Can you work these out from the drawing? Everything is in mm from the part's minimum corner. A direction names the side the tool comes from. Coordinates: 2 decimals unless noted, no trailing zeros. Write each loop counter-clockwise with the first axis right and the second up, starting at its lowest first coordinate (ties: lowest second). Pieces come first, ordered by that corner, then holes. Notation, with made-up numbers: M 11,79 L 16,79 A21 ccw 16,113 Z; hole C 56,56.5 d7. An arc over 180 degrees is marked long. Write item = value, one per line.
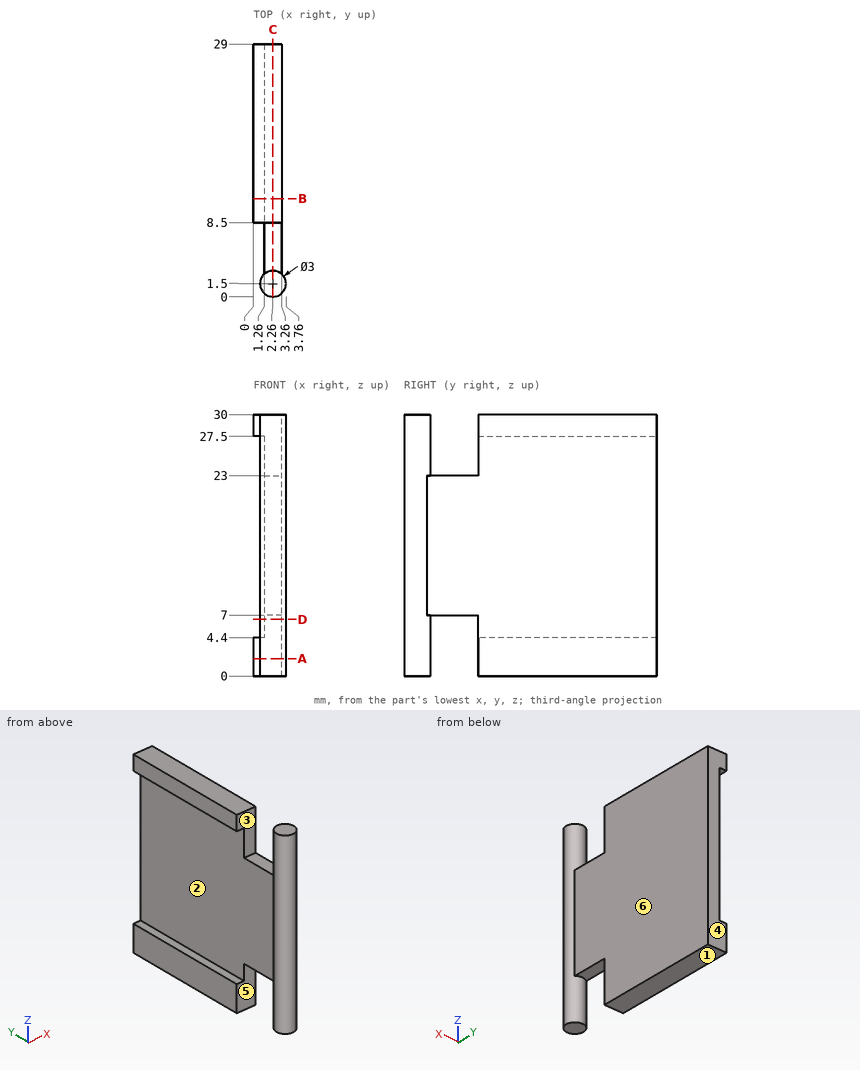
Item 1: Imagine slicing it at A-A (z = 2). Write out the boundary of the cut face in (x, y), and give its area (3 significant figures).
Numbers:
outline = M 0,8.5 L 3.26,8.5 L 3.26,29 L 0,29 Z; C 2.26,1.5 d3
area = 73.9 mm²
Item 2: If we mould it in two halves opening along Y, with no side actions, what happens to the marked faces 3, 4, 5 and 6? For each: pulls with the +Y half, pulls with the -Y half, needs draft (parallel to the pull), parting line crosses it, or undercut.
Numbers:
face_3 = undercut
face_4 = pulls with the +Y half
face_5 = undercut
face_6 = needs draft
Item 3: If I drill on line 1 along Z through (x, y) = (0.25, 15.25); line 2 along X through (y, z) = (14, 23.25); line 3 along X through (y, z) = (13, 4), over which ranges is the centre line in solid material (lowest first)?
Numbers:
line_1 = 0 to 4.4, 27.5 to 30
line_2 = 1.26 to 3.26
line_3 = 0 to 3.26
Item 4: Imagine slicing it at D-D (z = 6.5). Write out the boundary of the cut face in (x, y).
Numbers:
outline = C 2.26,1.5 d3; M 1.26,8.5 L 3.26,8.5 L 3.26,29 L 1.26,29 Z
Item 5: I'm going to push flat-ended pins straight in: P1, Ø3, axis at y = 9, z = 16.5, coming from the -X side; P2, Ø2, axis at x = 2, y = 5.5, coming from the -Z side; P3, Ø0.6, axis at x = 2, y = 7, coming from the +Z side. Where does each tip first touch, or does it pass through?
Numbers:
P1 = 1.26
P2 = 7
P3 = 23
Item 6: Imagine slicing it at B-B (y = 11.25). Write out the boundary of the cut face in (x, z), and give its area (3 significant figures).
Numbers:
outline = M 0,0 L 3.26,0 L 3.26,30 L 0,30 L 0,27.5 L 1.26,27.5 L 1.26,4.4 L 0,4.4 Z
area = 68.7 mm²
Item 7: Imagine slicing it at C-C (x = 2.26). Write out the boundary of the cut face in (y, z), and give its area (3 significant figures).
Numbers:
outline = M 0,0 L 3,0 L 3,7 L 8.5,7 L 8.5,0 L 29,0 L 29,30 L 8.5,30 L 8.5,23 L 3,23 L 3,30 L 0,30 Z
area = 793 mm²
Item 8: For the marked faces 1 and 2, which set-ups out of +Z, -Z, +X, -X, +Y, -Y let a thin tool reach every point of the face, with its end or its side?
Numbers:
face_1 = -Z, +X, -X, +Y, -Y
face_2 = -X, +Y
